from build123d import *

# Parameters (mm, degrees)
SKETCH1_R           = 1.25
SKETCH1_W           = 156.43
SKETCH1_H           = 89.15
BOSS_EXTRUDE1_DEPTH = 4
BOSS_EXTRUDE2_START = -6.1
SKETCH1_3_R         = 1.25
BOSS_EXTRUDE2_DEPTH = 6.1
FILLET1_R           = 4
SKETCH2_W           = 17.19
SKETCH2_H           = 6.1
CUT_EXTRUDE1_DEPTH  = 1
SKETCH3_W           = 6.1
SKETCH3_H           = 11.97
CUT_EXTRUDE2_DEPTH  = 1
SKETCH4_R           = 1.25
CUT_EXTRUDE3_DEPTH  = 125.056407333


with BuildPart() as part:
    # Sketch1 → Boss-Extrude1 (new body)
    with BuildSketch(Plane.XY):
        with BuildLine():
            Line((-98.129170507, 35.926013825), (-98.129170507, -67.223986175))
            ThreePointArc((-98.129170507, -67.223986175), (-95.786024756, -72.880840425), (-90.129170507, -75.223986175))
            Line((-90.129170507, -75.223986175), (80.300829493, -75.223986175))
            ThreePointArc((80.300829493, -75.223986175), (85.957683743, -72.880840425), (88.300829493, -67.223986175))
            Line((88.300829493, -67.223986175), (88.300829493, 35.926013825))
            ThreePointArc((88.300829493, 35.926013825), (85.957683743, 41.582868074), (80.300829493, 43.926013825))
            Line((80.300829493, 43.926013825), (-90.129170507, 43.926013825))
            ThreePointArc((-90.129170507, 43.926013825), (-95.786024756, 41.582868074), (-98.129170507, 35.926013825))
        make_face()
        with Locations((80.300829493, 35.926013825)):
            Circle(SKETCH1_R, mode=Mode.SUBTRACT)
        with Locations((80.300829493, -67.223986175)):
            Circle(SKETCH1_R, mode=Mode.SUBTRACT)
        with Locations((-90.129170507, -67.223986175)):
            Circle(SKETCH1_R, mode=Mode.SUBTRACT)
        with Locations((-90.129170507, 35.926013825)):
            Circle(SKETCH1_R, mode=Mode.SUBTRACT)
        with Locations((-4.914170507, -15.648986175)):
            Rectangle(SKETCH1_W, SKETCH1_H, mode=Mode.SUBTRACT)
    extrude(amount=BOSS_EXTRUDE1_DEPTH)

    # Sketch1<3> → Boss-Extrude2 (add)
    with BuildSketch(Plane.XY.offset(BOSS_EXTRUDE2_START)):
        with BuildLine():
            ThreePointArc((-90.129170507, 43.926013825), (-95.786024756, 41.582868074), (-98.129170507, 35.926013825))
            Line((-98.129170507, 35.926013825), (-98.129170507, -67.223986175))
            ThreePointArc((-98.129170507, -67.223986175), (-95.786024756, -72.880840425), (-90.129170507, -75.223986175))
            Line((-90.129170507, -75.223986175), (80.300829493, -75.223986175))
            ThreePointArc((80.300829493, -75.223986175), (85.957683743, -72.880840425), (88.300829493, -67.223986175))
            Line((88.300829493, -67.223986175), (88.300829493, 35.926013825))
            ThreePointArc((88.300829493, 35.926013825), (85.957683743, 41.582868074), (80.300829493, 43.926013825))
            Line((80.300829493, 43.926013825), (-90.129170507, 43.926013825))
        make_face()
        with Locations((-90.129170507, -67.223986175)):
            Circle(SKETCH1_3_R, mode=Mode.SUBTRACT)
        with Locations((80.300829493, -67.223986175)):
            Circle(SKETCH1_3_R, mode=Mode.SUBTRACT)
        with BuildLine():
            Line((-89.239170507, -64.383986175), (-89.239170507, 35.048289495))
            ThreePointArc((-89.239170507, 35.048289495), (-91.378326538, 35.97193996), (-89.177120088, 36.736013825))
            Line((-89.177120088, 36.736013825), (76.680829493, 36.736013825))
            Line((76.680829493, 36.736013825), (76.680829493, -64.383986175))
            Line((76.680829493, -64.383986175), (-89.239170507, -64.383986175))
        make_face(mode=Mode.SUBTRACT)
        with Locations((80.300829493, 35.926013825)):
            Circle(SKETCH1_3_R, mode=Mode.SUBTRACT)
    extrude(amount=BOSS_EXTRUDE2_DEPTH)

    # Fillet1
    fillet1_edges = [part.edges().sort_by_distance(p)[0] for p in [
        (-95.786024756, 41.582868074, 4),
        (-4.914170507, 43.926013825, 4),
        (85.957683743, 41.582868074, 4),
        (88.300829493, -15.648986175, 4),
        (85.957683743, -72.880840425, 4),
        (-4.914170507, -75.223986175, 4),
        (-95.786024756, -72.880840425, 4),
        (-4.914170507, -60.223986175, 4),
        (-4.914170507, 28.926013825, 4),
        (-83.129170507, -15.648986175, 4),
        (73.300829493, -15.648986175, 4),
        (-98.129170507, -15.648986175, 4),
    ]]
    fillet(fillet1_edges, radius=FILLET1_R - 0.0001)  # a hair under: the kernel refuses the full size

    # Sketch2 → Cut-Extrude1 (cut)
    with BuildSketch(Plane.XZ.offset(-36.736013825)):
        with Locations((-30.314170507, -3.05)):
            Rectangle(SKETCH2_W, SKETCH2_H)
    extrude(amount=-CUT_EXTRUDE1_DEPTH, mode=Mode.SUBTRACT)

    # Sketch3 → Cut-Extrude2 (cut)
    with BuildSketch(Plane.ZY.offset(-76.680829493)):
        with Locations((-3.05, -16.608986175)):
            Rectangle(SKETCH3_W, SKETCH3_H)
    extrude(amount=-CUT_EXTRUDE2_DEPTH, mode=Mode.SUBTRACT)

    # Sketch4 → Cut-Extrude3 (cut, through all)
    with BuildSketch(Plane(origin=(0, 0, -6.1), x_dir=(-1, 0, 0), z_dir=(0, 0, -1))):
        with Locations((4.909170507, 40.776013825)):
            Circle(SKETCH4_R)
        with Locations((-80.300829493, -15.243986175)):
            Circle(SKETCH4_R)
        with Locations((4.909170507, -67.223986175)):
            Circle(SKETCH4_R)
        with Locations((90.129170507, -3.883986175)):
            Circle(SKETCH4_R)
    extrude(amount=-CUT_EXTRUDE3_DEPTH, mode=Mode.SUBTRACT)


solid = part.part
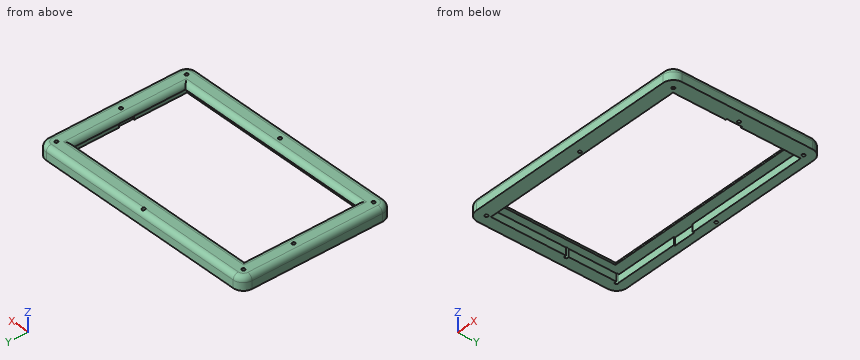
Can you work these out from the model? Positions are in its coordinate system, mm. Coordinates: 2 decimals unless noted, no trailing zeros. Order: outer loops, then holes, each group sorted by start corner. A loop starts at its lowest first (then second) coordinate and runs counter-clockwise, first axis right, second up. Notation, with made-up numbers: (56.25, 45.25) -> (95.25, 45.25) arc R14 cw to (95.25, 64.25) -> close; hole circle Ø11 at (47, 19). An arc over 180 degrees is marked (long way). Use one line per item in the form item = value.
Q1. Imagine slicing it at D-D, the plane y = 31. List the corners of the cut face in (x, z) for me.
From the geometry:
outline = (-98.13, -6.1) -> (-89.24, -6.1) -> (-89.24, 0) -> (76.68, 0) -> (76.68, -6.1) -> (88.3, -6.1) -> (88.3, 0) arc R4 ccw to (84.3, 4) -> (77.3, 4) arc R4 ccw to (75.37, 3.51) -> (-85.2, 3.51) arc R4 ccw to (-87.13, 4) -> (-94.13, 4) arc R4 ccw to (-98.13, 0) -> close
Q2. Imagine slicing it at C-C, the plane z = -4.5. Give the number of separate pieces and of enclosed holes in the cut face, then the cut area to 3 significant figures.
From the geometry:
separate_pieces = 1
enclosed_holes = 7
area = 5,310 mm²
Q3. I need wall thicknesses on L1, parallel to Y at x = -5, z = -3.5; L2, parallel to Y at x = 4.5, z = 0.25; L3, parallel to X at y = -28.5, z = -1. Which ranges of each line are inside material? Lowest first, please.
From the geometry:
L1 = -75.22 to -68.47, -65.98 to -64.38, 36.74 to 39.53, 42.02 to 43.93
L2 = -75.22 to -60.23, 28.93 to 43.92
L3 = -98.13 to -89.24, 76.68 to 88.3
Q4. Will these pins go through, and if not, where does the flat tip stop? P1, Ø1.1, axis at y = 37, z = -2.5, coming from the -X side; P2, Ø0.5, axis at y = 37, z = -4, coming from the +X side.
From the geometry:
P1 = -98.11
P2 = 88.26
